from build123d import *

# Parameters (mm, degrees)
F0_W     = 42.8625
F0_H     = 42.8625
F0_R     = 10.31875
F1_DEPTH = 40.64
F3_DEPTH = 42.8635
F4_R     = 0.508


with BuildPart() as f1:
    # F0 (on Front) → F1 (new body)
    with BuildSketch(Plane.XZ):
        with Locations((21.43125, -21.43125)):
            Rectangle(F0_W, F0_H)
        with Locations((21.43125, -21.43125)):
            Circle(F0_R, mode=Mode.SUBTRACT)
    extrude(amount=F1_DEPTH)

    # F2 (on face) → F3 (cut, through all)
    with BuildSketch(Plane.YZ.offset(42.8625)):
        Polygon((0, -42.8625), (-40.64, 0), (-40.64, -42.8625), align=None)
    extrude(amount=-F3_DEPTH, mode=Mode.SUBTRACT)

    # F4
    f4_edges = [f1.edges().sort_by_distance(p)[0] for p in [
        (42.8625, 0, -21.43125),
        (42.8625, -20.32, 0),
        (42.8625, -20.32, -21.43125),
        (21.43125, 0, -42.8625),
        (21.43125, -40.64, 0),
        (0, -20.32, -21.43125),
        (11.1125, -20.317825, -21.433544),
        (0, 0, -21.43125),
        (0, -20.32, 0),
        (21.43125, 0, 0),
    ]]
    fillet(f4_edges, radius=F4_R)


solid = f1.part
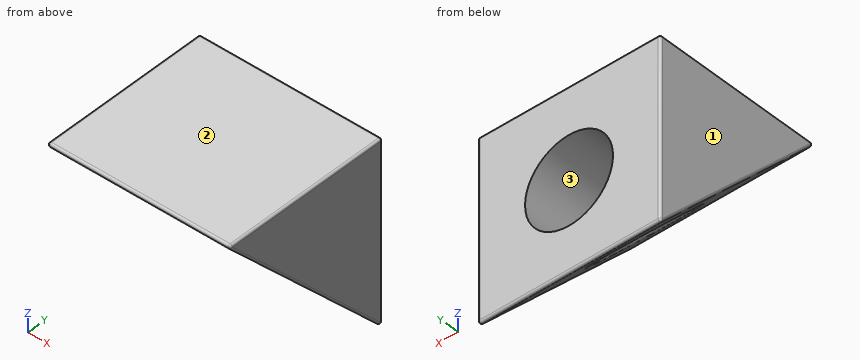
Verification items for the finished model (mm, model axes). Face numbers are marked on the shaded views. Round coordinates to 2 decimals unless told otherwise and drop trailing zeros. Write each loop counter-clockwise with the first axis right and the second up, starting at its lowest first coordinate (ties: lowest second). Pieces come first, ordered by that corner, then holes.
(1) Depth check by flat-ended pin: pin 1 Ø18.5 at (x, z) = (21.43, -21.43) entering from -Y; pin 2 Ø6 at (x, y) = (21.5, -18) entering from -Z; pin 3 Ø1.5 at (x, y) = (11, -25.5) entering from -Z; pin 4 Ø1.5 at (x, y) = (13.5, -19) entering from -Z. Enter the tip coordinate at first touch or a pass-through.
Returned:
pin 1: passes through
pin 2: stops at z = -11.58
pin 3: stops at z = -16.76
pin 4: stops at z = -15.85
(2) Mould release check, pull along X, two halves, no side actions. Record for the marked faces 1, 2 and 3: pulls with the +X half, pulls with the -X half, needs draft (parallel to the pull), parting line crosses it, or undercut.
Returned:
face 1: pulls with the -X half
face 2: needs draft
face 3: undercut
(3) Material ranges on line 1 (X direction, y = -20, z = -18.5); line 2 (Z direction, x = 20, y = -3.5); line 3 (X direction, y = -2, z = -20), recorded low to high.
Returned:
line 1: x = 0 to 11.54, 31.32 to 42.86
line 2: z = -39.17 to -31.65, -11.21 to 0
line 3: x = 0 to 11.21, 31.65 to 42.86
(4) Section check A-A (x = 4). Enter the section's corners in (y, z), plus the area to 3 significant figures.
Returned:
outline: (-39.83, -0.86) - (-0.88, -41.94) arc R0.51 ccw to (0, -41.59) - (0, -0.51) arc R0.51 ccw to (-0.51, 0) - (-39.46, 0) arc R0.51 ccw to start
area: 870 mm2
